Could you check a few things on this model? Use its own coordinates, in mm. A direction names the side the tool comes from. Coordinates: 2 decimals unless noted, no trailing zeros. Loops run counter-clockwise (first coordinate to the right, second up) from the corner with the lowest first, then second, coordinate; pieces in that order, holes last.
from build123d import *

# Parameters (mm, degrees)
EXTRUDE_1_DEPTH     = 40
SKETCH_3_R          = 2.5
CUT_EXTRUDE_2_DEPTH = 35
SKETCH_4_OUTSIDE_W  = 36.852
SKETCH_4_OUTSIDE_H  = 40.564
SKETCH_4_OUTSIDE_R  = 8
CUT_EXTRUDE_3_DEPTH = 10
SKETCH_5_R          = 5
CUT_EXTRUDE_4_DEPTH = 15


with BuildPart() as part:
    # Эскиз1 → Бобышка-Вытянуть1 (new body)
    with BuildSketch(Plane(origin=(0, 0, 0), x_dir=(1, 0, 0), z_dir=(0, 1, 0))):
        Polygon((0, 13.856406461), (-12, 6.92820323), (-12, -6.92820323), (0, -13.856406461), (12, -6.92820323), (12, 6.92820323), align=None)
    extrude(amount=EXTRUDE_1_DEPTH)

    # Эскиз3 → Вырез-Вытянуть2 (cut)
    with BuildSketch(Plane(origin=(0, 40, 0), x_dir=(1, 0, 0), z_dir=(0, 1, 0))):
        Circle(SKETCH_3_R)
    extrude(amount=-CUT_EXTRUDE_2_DEPTH, mode=Mode.SUBTRACT)

    # Эскиз4 outside → Вырез-Вытянуть3 (cut)
    with BuildSketch(Plane(origin=(0, 40, 0), x_dir=(1, 0, 0), z_dir=(0, 1, 0))):
        Rectangle(SKETCH_4_OUTSIDE_W, SKETCH_4_OUTSIDE_H)
        Circle(SKETCH_4_OUTSIDE_R, mode=Mode.SUBTRACT)
    extrude(amount=-CUT_EXTRUDE_3_DEPTH, mode=Mode.SUBTRACT)

    # Эскиз5 → Вырез-Вытянуть4 (cut)
    with BuildSketch(Plane(origin=(-6, 0, -10.392304845), x_dir=(-0.866025404, 0, 0.5), z_dir=(-0.5, 0, -0.866025404))):
        with Locations((0, 8)):
            Circle(SKETCH_5_R)
    extrude(amount=-CUT_EXTRUDE_4_DEPTH, mode=Mode.SUBTRACT)


solid = part.part
(1) Imagine slicing it at B-B, the plane y = 7.5. Write out the boundary of the cut face in (x, z).
Answers:
outline: (-12, -6.93) - (-10.31, -7.9) - (-2.81, 5.09) - (5.81, 0.11) - (-1.69, -12.88) - (0, -13.86) - (12, -6.93) - (12, 6.93) - (0, 13.86) - (-12, 6.93) - close
(2) I need wall thicknesses on probe 1 along Z at (x, y) = (0, 26); probe 2 along X at (y, z) = (20.5, 0); probe 3 along Z at (x, y) = (0, 34.25). Which ranges of each line are inside material? Lowest first, please.
Answers:
probe 1: z = -13.86 to -2.5, 2.5 to 13.86
probe 2: x = -12 to -2.5, 2.5 to 12
probe 3: z = -8 to -2.5, 2.5 to 8
(3) Imagine slicing it at C-C, the plane x = 6.75. Write out the boundary of the cut face in (y, z).
Answers:
outline: (0, -9.96) - (30, -9.96) - (30, -4.29) - (40, -4.29) - (40, 4.29) - (30, 4.29) - (30, 9.96) - (0, 9.96) - close
(4) Imagine slicing it at A-A, the plane y = 17.5. Write out the boundary of the cut face in (x, z), and give its area (3 significant figures).
Answers:
outline: (-12, -6.93) - (0, -13.86) - (12, -6.93) - (12, 6.93) - (0, 13.86) - (-12, 6.93) - close; hole circle Ø5 at (0, 0)
area: 479 mm2
(5) Which directions (+Z, -Z, +X, -X, +Y, -Y) give clear straight access to the entire face, cutting with the end or side of a thin tool? Please do faces 4 (the face through (0, 0, 0)), 5 (the face through (-0.54, 26.36, 2.44)), 6 (the face through (1.561, 8.07, 2.563)).
Answers:
face 4: +Z, -Z, +X, -X, -Y
face 5: +Y
face 6: none
(6) For pin 1 (4 mm diameter, centred on x = -9.5, z = -3.5, fed in from +Y); pin 2 (3 mm diameter, centred on x = 4, z = -1.5, fed in from -Y); pin 3 (12 mm diameter, centred on x = 0.5, y = 8.5, fed in from +Z); pin 4 (10 mm diameter, centred on x = -8.5, y = 21, fed in from +Z), each with a flat end and sliding along its axis, tell me the tip position at first contact or that it passes through.
Answers:
pin 1: stops at y = 30
pin 2: stops at y = 0
pin 3: stops at z = 13.86
pin 4: stops at z = 11.84
(7) We'd pull the mould along Z, two halves only. Please class faces 1 (the face through (-12, 15, 0)), 2 (the face through (5.92, 14.79, 10.44)), 3 (the face through (-1.36, 3.12, -4.53)): +Z half, -Z half, draft (parallel to the pull), parting line (faces both ways), or undercut.
Answers:
face 1: draft
face 2: +Z half
face 3: undercut
(8) Imagine slicing it at D-D, the plane z = 11.75. Write out the boundary of the cut face in (x, y).
Answers:
outline: (-3.65, 0) - (3.65, 0) - (3.65, 30) - (-3.65, 30) - close
